Source: CAD feature listing. Evaluate the final solid. Frame: model axes, mm. A direction names the side the tool comes from. Coordinates: 2 decimals unless noted, no trailing zeros. Order: outer loops, then holes, each group sorted by start corner. A loop starts at its lowest first (then second) coordinate and runs counter-clockwise, first axis right, second up.
```python
from build123d import *

# Parameters (mm, degrees)
F0_R     = 2.35
F0_R_2   = 1.5
F1_DEPTH = 3.6
F2_DEPTH = 0.4
F3_DEPTH = 2.5
F4_R     = 0.5
F5_DEPTH = 0.3
F6_R     = 0.225
F7_DEPTH = 5


with BuildPart() as f1:
    # F0 (on Top) → F1 (new body)
    with BuildSketch(Plane.XY):
        Circle(F0_R)
        Circle(F0_R_2, mode=Mode.SUBTRACT)
    extrude(amount=F1_DEPTH)

    # F0 (on Top) → F2 (join)
    with BuildSketch(Plane.XY):
        with BuildLine():
            Line((2.262742, 2.969848), (1.522613, 2.22972))
            ThreePointArc((1.522613, 2.22972), (-1.909188, -1.909188), (2.22972, 1.522613))
            Line((2.22972, 1.522613), (2.969848, 2.262742))
            Line((2.969848, 2.262742), (2.616295, 2.616295))
            Line((2.616295, 2.616295), (2.262742, 2.969848))
        make_face()
        Circle(F0_R, mode=Mode.SUBTRACT)
    extrude(amount=F2_DEPTH)

    # F0 (on Top) → F3 (join)
    with BuildSketch(Plane.XY):
        Circle(F0_R_2)
    extrude(amount=F3_DEPTH)

    # F4 (on face) → F5 (join)
    with BuildSketch(Plane.XY.offset(2.5)):
        with Locations((0, -0.282093)):
            Circle(F4_R)
    extrude(amount=F5_DEPTH)

    # F6 (on face) → F7 (join)
    with BuildSketch(Plane.XY):
        with Locations((0, -1.27)):
            Circle(F6_R)
        with Locations((-1.27, 0)):
            Circle(F6_R)
        with Locations((0, 1.27)):
            Circle(F6_R)
    extrude(amount=-F7_DEPTH)


solid = f1.part
```
1. Draft query along X for faces 1 (the flat face through (2, 2, 0.4)), 2 (the cylindrical face through (-1.5, 0.07, 3.04)), 3 (the cylindrical face through (-0.509, -2.294, 1.978)). Return one class per face: +X half, -X half, draft (parallel to the pull), parting line (faces both ways), or undercut.
2. Contact query for flat-ended pins moving along their axis: P1, Ø1.5, axis at y = 0, z = -2, coming from the +X side (3 decimals); P2, Ø3, axis at x = 0.5, z = -3, coming from the +Y side (3 decimals); P3, Ø3, axis at x = -1.5, y = -1.5, coming from the -Z side; P4, Ø0.9, axis at x = 0, y = 0.5, coming from the +Z side. Output: stop coordinate, or through.
3. Section query C-C, the plane z = -3.25. Output: boundary loops of the cut face in (x, y) (3 decimals).
4. Access query for faces 4 (the flat face through (0, 0, 0)), 5 (the cylindrical face through (-1.987, -1.829, 0.197)), 6 (the flat face through (0, 0, 2.8)). Directions: +Z, -Z, +X, -X, +Y, -Y. A direction counts if a zero-diameter tool reaches every point of the face in a straight line with its end or side. Return the directions, or none.
5. Section query A-A, the plane x = 0. Output: boundary loops of the cut face in (y, z) (3 decimals), plus the area to 3 significant figures.
6. Section query B-B, the plane x = 2.5. Output: boundary loops of the cut face in (y, z), plus the area to 3 significant figures.
7. Section query D-D, the plane y = 0.95. Output: boundary loops of the cut face in (x, z), plus the area to 3 significant figures.
8. Material intervals for line 1 along Z through (x, y) = (-1.65, -0.4); line 2 along Y through (x, z) = (0, 2.95); line 3 along Z through (x, y) = (2.5, 0.75), sorted ascending.
Answer key:
1. face 1: draft
1. face 2: undercut
1. face 3: parting line
2. P1: stops at x = -1.045
2. P2: stops at y = 1.495
2. P3: stops at z = -5
2. P4: stops at z = 2.8
3. outline: circle Ø0.45 at (-1.27, 0); circle Ø0.45 at (0, -1.27); circle Ø0.45 at (0, 1.27)
4. face 4: -Z
4. face 5: +Z, -Z
4. face 6: +Z
5. outline: (-2.7, 0) - (-1.495, 0) - (-1.495, -5) - (-1.045, -5) - (-1.045, 0) - (1.045, 0) - (1.045, -5) - (1.495, -5) - (1.495, 0) - (2.7, 0) - (2.7, 0.4) - (2.35, 0.4) - (2.35, 3.6) - (1.5, 3.6) - (1.5, 2.5) - (0.218, 2.5) - (0.218, 2.8) - (-0.782, 2.8) - (-0.782, 2.5) - (-1.5, 2.5) - (-1.5, 3.6) - (-2.35, 3.6) - (-2.35, 0.4) - (-2.7, 0.4) - close
5. area: 18.7 mm2
6. outline: (-1.02, 0) - (1.02, 0) - (1.02, 0.4) - (-1.02, 0.4) - close; (1.79, 0) - (2.73, 0) - (2.73, 0.4) - (1.79, 0.4) - close
6. area: 1.19 mm2
7. outline: (-2.53, 0) - (2.53, 0) - (2.53, 0.4) - (2.15, 0.4) - (2.15, 3.6) - (1.16, 3.6) - (1.16, 2.5) - (-1.16, 2.5) - (-1.16, 3.6) - (-2.15, 3.6) - (-2.15, 0.4) - (-2.53, 0.4) - close
7. area: 13.2 mm2
8. line 1: z = 0 to 3.6
8. line 2: y = -2.35 to -1.5, 1.5 to 2.35
8. line 3: z = 0 to 0.4
